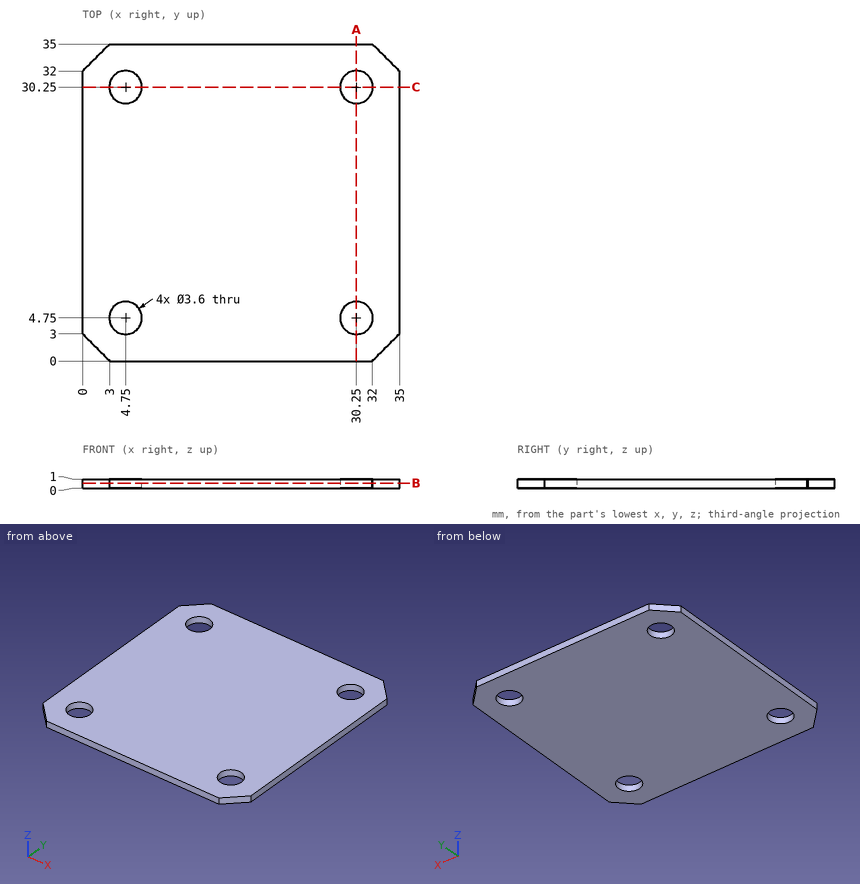
Check sheet for the drawn part. Datum: minimum x, y, z corner. Units: mm. Coordinates: 2 decimals unless noted, no trailing zeros. Loops run counter-clockwise (first coordinate to the right, second up) from the corner with the lowest first, then second, coordinate; pieces in that order, holes last. Notation, with made-up numbers: (-34.75, 22.5) - (18.25, 22.5) arc R12 ccw to (18.25, 42.5) - close; hole circle Ø11 at (-16.5, 36). An arc over 180 degrees is marked (long way). Put each result on its own line as item: value.
Item 1: Section check A-A (x = 30.25). Enter the section's corners in (y, z).
Conclusion:
outline: (0, 0) - (2.95, 0) - (2.95, 1) - (0, 1) - close; (6.55, 0) - (28.45, 0) - (28.45, 1) - (6.55, 1) - close; (32.05, 0) - (35, 0) - (35, 1) - (32.05, 1) - close
Item 2: Scan lines: line 1 along Y through (x, z) = (30.25, 0.5); line 2 along X through (y, z) = (30.5, 0.2); line 3 along Y through (x, z) = (31, 0.7). Record each from-to range of solid material in increasing order.
Conclusion:
line 1: y = 0 to 2.95, 6.55 to 28.45, 32.05 to 35
line 2: x = 0 to 2.97, 6.53 to 28.47, 32.03 to 35
line 3: y = 0 to 3.11, 6.39 to 28.61, 31.89 to 35
Item 3: Section check B-B (z = 0.55). Enter the section's corners in (x, y), then the cut area to 3 significant figures.
Conclusion:
outline: (0, 3) - (3, 0) - (32, 0) - (35, 3) - (35, 32) - (32, 35) - (3, 35) - (0, 32) - close; hole circle Ø3.6 at (4.75, 4.75); hole circle Ø3.6 at (4.75, 30.25); hole circle Ø3.6 at (30.25, 4.75); hole circle Ø3.6 at (30.25, 30.25)
area: 1,170 mm2
